The model under review builds one solid part; all positions refer to its coordinate system, in mm. Coordinates: 2 decimals unless noted, no trailing zeros. Loops run counter-clockwise (first coordinate to the right, second up) from the corner with the lowest first, then second, coordinate; pieces in that order, holes last. Notation, with made-up numbers: (-5.75, 86.25) - (4.25, 86.25) arc R29 ccw to (4.25, 121.25) - close; hole circle Ø11 at (-18.5, 63.5). An arc over 180 degrees is marked (long way). One line per item, written item: value. Start each with the question number.
1. Insertion check: P1, Ø4, axis at y = -15, z = 0, coming from the +X side; P2, Ø1, axis at x = -4, y = -11.5, coming from the +Z side; P3, Ø5, axis at x = 1, z = -5.5, coming from the +Y side; P4, Ø1.5, axis at x = -3, z = 3, coming from the -Y side. Each pin has a flat end and moves straight along its axis. Give the tip position at first contact, or say it passes through.
2. We need section C-C, the plane y = -4.25. Give the boundary of the cut face in (x, z), then the cut area to 3 significant figures.
3. To check wall thickness, follow line 1 (Z direction, x = -0.25, y = -11); line 2 (X direction, y = -14, z = -3); line 3 (Z direction, x = -4.5, y = -1.75). State the ranges of each line that lie inside material, in increasing order.
4. Mouldability with a two-part tool opening along Y and no side actions: class faces 1 (the face through (3.905, -8.507, 0.867)), 2 (the face through (0, -20, 0)), 3 (the face through (0, -15, 5)) as +Y half, -Y half, draft (parallel to the pull), parting line (faces both ways), or undercut.
5. We need section D-D, the plane y = -12.5. Give the boundary of the cut face in (x, z), then the cut area to 3 significant figures.
from build123d import *

# Parameters (mm, degrees)
CHAMFER_1_SIZE = 1


with BuildPart() as part:
    # 草图1 → 旋转1 (revolve)
    with BuildSketch(Plane.XY, mode=Mode.PRIVATE) as revolve_1_sk:
        with BuildLine():
            Line((8, -2.143593539), (8, -8))
            Line((8, -8), (4, -8))
            Line((4, -8), (4, -9))
            Line((4, -9), (5, -9))
            Line((5, -9), (5, -20))
            Line((5, -20), (0, -20))
            Line((0, -20), (0, 0))
            ThreePointArc((0, 0), (4.141104722, -0.545186779), (8, -2.143593539))
        make_face()
    revolve(revolve_1_sk.sketch.rotate(Axis((0, -20, 0), (0, 1, 0)), 90), axis=Axis((0, -20, 0), (0, 1, 0)))

    # 倒角1
    chamfer_1_edges = [part.edges().sort_by_distance(p)[0] for p in [
        (0, -9, 5),
        (0, -20, 5),
    ]]
    chamfer(chamfer_1_edges, length=CHAMFER_1_SIZE - 0.0001)  # a hair under: the kernel refuses the full size


solid = part.part
Findings below:
1. P1: x = 5
1. P2: z = 3.57
1. P3: y = -0.3
1. P4: y = -20
2. outline: circle Ø16 at (0, 0)
2. area: 201 mm2
3. line 1: -4.99 to 4.99
3. line 2: -4 to 4
3. line 3: -5.72 to 5.72
4. face 1: undercut
4. face 2: -Y half
4. face 3: draft
5. outline: circle Ø10 at (0, 0)
5. area: 78.5 mm2
